from build123d import *

# Parameters (mm, degrees)
M3X0_5_TAPPED_HOLE2_D   = 2.5
M3X0_5_TAPPED_HOLE3_D   = 2.5
CUT_EXTRUDE4_DEPTH      = 49.457559
CIRPATTERN3_COUNT       = 4
CIRPATTERN4_COUNT       = 6
CHAMFER1_SIZE           = 0.5
CUT_EXTRUDE6_DEPTH      = 49.457559
CUT_EXTRUDE6_DEPTH_BACK = 49.457559
CUT_EXTRUDE7_START      = -6.4
SKETCH18_W              = 13.80373
SKETCH18_H              = 8
CUT_EXTRUDE7_DEPTH      = 43.057559


with BuildPart() as part:
    # Sketch1 → Revolve1 (revolve)
    with BuildSketch(Plane.XY, mode=Mode.PRIVATE) as revolve1_sk:
        Polygon((-11.9, 4), (-11.9, -4), (-12.9, -4), (-12.9, -8), (-31.15, -8), (-31.15, 1), (-31.9, 1), (-31.9, 4), (-32.65, 4), (-32.65, -14.2), (-32.15, -14.7), (-27.65, -14.7), (-27.65, -9.5), (-24.5, -9.5), (-24.5, -12.5), (-19.5, -12.5), (-19.5, -9.5), (-10.9, -9.5), (-10.9, -6.4), (-8.5, -6.4), (-8.5, -5.4), (-9, -5.4), (-9, 4), align=None)
    revolve(revolve1_sk.sketch.rotate(Axis((0, 0, 0), (0, 1, 0)), 270), axis=Axis((0, 0, 0), (0, 1, 0)))

    # M3x0.5 Tapped Hole2 (through all)
    with Locations(Plane(origin=(0, -14.7, 0), x_dir=(-1, 0, 0), z_dir=(0, -1, 0))):
        with Locations((0, 30)):
            m3x0_5_tapped_hole2 = Hole(M3X0_5_TAPPED_HOLE2_D / 2)

    # M3x0.5 Tapped Hole3 (through all)
    with Locations(Plane(origin=(0, -12.5, 0), x_dir=(-1, 0, 0), z_dir=(0, -1, 0))):
        with Locations((-15.5, 15.5), (15.5, 15.5), (-15.5, -15.5), (15.5, -15.5)):
            Hole(M3X0_5_TAPPED_HOLE3_D / 2)

    # Sketch13 → Cut-Extrude4 (cut, through all)
    with BuildSketch(Plane(origin=(0, 0, 0), x_dir=(1, 0, 0), z_dir=(0, 1, 0))):
        with BuildLine():
            Line((14.252286, 19.889192), (4.79293, 12.853907))
            ThreePointArc((4.79293, 12.853907), (3.992298, 12.497696), (3.116234, 12.517951))
            ThreePointArc((3.116234, 12.517951), (0, 12.9), (-3.116234, 12.517951))
            ThreePointArc((-3.116234, 12.517951), (-3.992298, 12.497696), (-4.79293, 12.853907))
            Line((-4.79293, 12.853907), (-14.252286, 19.889192))
            ThreePointArc((-14.252286, 19.889192), (-15.056541, 21.587496), (-14.097195, 23.203267))
            ThreePointArc((-14.097195, 23.203267), (0, 27.15), (14.097195, 23.203267))
            ThreePointArc((14.097195, 23.203267), (15.056541, 21.587496), (14.252286, 19.889192))
        make_face()
    cut_extrude4 = extrude(amount=-CUT_EXTRUDE4_DEPTH, mode=Mode.SUBTRACT)

    # CirPattern3: Cut-Extrude4 ×4 about axis
    cirpattern3_axis = Axis((0, 0, 0), (0, 1, 0))
    for i in range(1, CIRPATTERN3_COUNT):
        add(cut_extrude4.rotate(cirpattern3_axis, i * 360 / CIRPATTERN3_COUNT), mode=Mode.SUBTRACT)

    # CirPattern4: M3x0.5 Tapped Hole2 ×6 about axis
    cirpattern4_axis = Axis((0, 0, 0), (0, 1, 0))
    for i in range(1, CIRPATTERN4_COUNT):
        add(m3x0_5_tapped_hole2.rotate(cirpattern4_axis, i * 360 / CIRPATTERN4_COUNT), mode=Mode.SUBTRACT)

    # Chamfer1
    chamfer1_edges = [part.edges().sort_by_distance(p)[0] for p in [
        (0, 4, 11.9),
        (0, -14.7, 27.65),
        (0, 4, 9),
    ]]
    chamfer(chamfer1_edges, length=CHAMFER1_SIZE)

    # Sketch16 → Cut-Extrude6 (cut, two sides: drawn at the far end of the back side and taken through both)
    with BuildSketch(Plane(origin=(0, 0, 0), x_dir=(1, 0, 0), z_dir=(0, 1, 0)).offset(-CUT_EXTRUDE6_DEPTH_BACK)):
        with BuildLine():
            Line((-18.769737, 4), (-11, 4))
            ThreePointArc((-11, 4), (-10.292893, 3.707107), (-10, 3))
            Line((-10, 3), (-10, -3))
            ThreePointArc((-10, -3), (-10.292893, -3.707107), (-11, -4))
            Line((-11, -4), (-18.769737, -4))
            ThreePointArc((-18.769737, -4), (-19.476844, -3.707107), (-19.769737, -3))
            Line((-19.769737, -3), (-19.769737, 3))
            ThreePointArc((-19.769737, 3), (-19.476844, 3.707107), (-18.769737, 4))
        make_face()
    extrude(amount=CUT_EXTRUDE6_DEPTH + CUT_EXTRUDE6_DEPTH_BACK, mode=Mode.SUBTRACT)

    # Sketch18 → Cut-Extrude7 (cut, through all)
    with BuildSketch(Plane(origin=(0, 0, 0), x_dir=(1, 0, 0), z_dir=(0, 1, 0)).offset(CUT_EXTRUDE7_START)):
        with Locations((-11.236069, 0)):
            Rectangle(SKETCH18_W, SKETCH18_H)
    extrude(amount=-CUT_EXTRUDE7_DEPTH, mode=Mode.SUBTRACT)


solid = part.part
Input: part model. Units: mm. Frame: model coordinates. A direction names the side the tool comes from. Give positions to 0.01 mm unless a question says otherwise; leave off trailing zeros. Answer as a JSON object with one key per item and string values. Group by question number.
Q1. Set-up query: faces 1 (the face through (4.8, -6.4, 7.2)), 2 (the face through (4, -8.7, -12.5)), 3 (the face through (6.9, 1, 30.6)). Return all of +Z, -Z, +X, -X, +Y, -Y with unobstructed straight access to the full face (end or side cutting, diameter ignored); none if empty.
Q2. Cut plane A-A, the plane z = 0. Count the separate pieces of the cut face and the enclosed holes in it, then the cut area to 3 significant figures.
Q3. Line query: probe 1 along X at (y, z) = (2.4, 0); probe 2 along X at (y, z) = (-5.55, 0); probe 3 along Z at (x, y) = (19, -10). Output: solid intervals per line, ascending.
Q4. First-contact query: pin 1 Ø11 at (x, z) = (-15, 14.5) entering from -Y; pin 2 Ø2 at (x, z) = (15.5, 15.5) entering from +Y; pin 3 Ø12 at (x, z) = (-17, 14) entering from -Y; pin 4 Ø8 at (x, y) = (24.5, -13) entering from +Z. Flat tips, straight axial feed; report the tip coordinate or a pass-through.
Results:
{
 "1": {"face 1": "-Y", "face 2": "+Y, -Y", "face 3": "+Y"},
 "2": {"separate pieces": "4", "enclosed holes": "0", "area": "149 mm^2"},
 "3": {"probe 1": "-32.65 to -31.9, -10 to -9, 9 to 11.9, 31.9 to 32.65", "probe 2": "-32.65 to -31.15, -10 to -8.5, 8.5 to 12.9, 31.15 to 32.65", "probe 3": "-26.55 to -20.09, -15.47 to -13.06, 13.06 to 15.47, 20.09 to 26.55"},
 "4": {"pin 1": "y = -12.5", "pin 2": "through", "pin 3": "y = -14.57", "pin 4": "z = 25.41"}
}
